Can you work these out from the model? Positions are in its coordinate system, mm. A direction names the side the tool comes from. Give positions to 0.01 mm unless a question says otherwise; leave off trailing zeros. Order: outer loops, then holes, each group sorted by start corner. A loop starts at its lowest first (then second) coordinate and runs counter-clockwise, first axis right, second up. Notation, with made-up numbers: M -16.75,-23 L 23.25,-23 A20 cw 23.25,-7 Z; hole C 28.25,-24.5 d1. An arc over 180 degrees is marked long. Use a Markdown table: item, result. Add a question column.
Autodesk Inventor part; units mm, degrees
ref_plane "YZ Plane" through (0, 0, 0) normal (1, 0, 0) x (0, 1, 0)
ref_plane "XZ Plane" through (0, 0, 0) normal (0, 1, 0) x (-1, 0, 0)
ref_plane "XY Plane" through (0, 0, 0) normal (0, 0, 1) x (1, 0, 0)
sketch "Sketch1" plane through (0, 0, 0) normal (0, 0, 1) x (1, 0, 0)
  line L0 (0, 0) -> (-184.15, 0)
  line L1 (-184.15, 0) -> (-184.15, 101.6)
  line L2 (-184.15, 101.6) -> (0, 101.6)
  line L3 (0, 101.6) -> (0, 0)
  dimension "d0" = 184.15
  dimension "d1" = 101.6
extrude "Extrusion1" add sketch "Sketch1" along normal blind 1.5875
chamfer "Chamfer1" distance 1.5875 angle 45 1 edges at (-184.15, 50.8, 0)
sketch "Sketch2" plane through (-184.15, 0, 1.5875) normal (-0.7071, 0, -0.7071) x (-0.7071, 0, 0.7071)
  line L0 (0, 101.6) -> (0, 0)
  line L1 (-2.2451, 101.6) -> (-2.2451, 0)
  line L2 (0, 101.6) -> (-2.2451, 101.6)
  line L3 (-2.2451, 0) -> (0, 0)
  point P0 (-131.3362, 0)
extrude "Extrusion2" add sketch "Sketch2" along normal blind 19.05
sketch "Sketch3" plane through (0, 0, 1.5875) normal (0, 0, 1) x (1, 0, 0)
  circle A0 centre (-19.05, 69.85) radius 2.1844
  line L0 (-184.15, 0) -> (0, 0)
  line L1 (-184.15, 101.6) -> (-184.15, 0)
  circle A1 centre (-171.45, 69.85) radius 2.1844
  point P0 (-231.8428, 57.2075)
  point P1 (-184.15, 46.6344)
  point P2 (-184.15, 42.2656)
  dimension "d9" = 4.3688
  dimension "d10" = 69.85
  dimension "d11" = 165.1
  dimension "d17" = 4.3688
  dimension "d18" = 152.4
extrude "Extrusion3" cut sketch "Sketch3" against normal blind 19.05
properties part number "frontwing"
1. On a 3-axis mill with a long thin cutter (end or side, diameter ignored), from which of +Z, -Z, +X, -X, +Y, -Y can I reach the whole of each face in a straight line? I mean faces 5 (the face through (-93, 52, 0)), 6 (the face through (-105, 0, 1)). Say none if no direction works.
2. If we section it at D-D, the plane x = -54.5: List the corners of the cut face in (y, z) for me.
3. If we section it at B-B, the plane y = 69.85: State how many separate pieces and enclosed holes the cut face has, then the cut area to 3 significant figures.
4. We'd pull the mould along Y, two halves only. Please class faces 1 (the face through (-190.79, 51.51, -5.05)), 2 (the face through (-173.632, 69.946, 0.805)), 3 (the face through (-113, 101.6, 1)), 4 (the face through (-18.042, 67.912, 0.805)): +Y half, -Y half, draft (parallel to the pull), parting line (faces both ways), or undercut.
5. I need wall thicknesses on L1, parallel to Y at x = -19.05, z = 1; L2, parallel to Z at x = -107, y = 62; L3, parallel to X at y = 46, z = -4.25. Which ranges of each line are inside material? Lowest first, please. Write a range as [from, to].
6. Will these pins go through, and if not, where does the flat tip stop? pin 1 (5 mm diameter, centred on x = -164, y = 75, fed in from -Z); pin 2 (5 mm diameter, centred on y = 20, z = -3.5, fed in from -X).
7. If we section it at A-A, the plane x = -171.45: List the corners of the cut face in (y, z) for me.
Geometry results:
| question | item | result |
|---|---|---|
| 1 | face 5 | -Z, +X, +Y, -Y |
| 1 | face 6 | +Z, -Z, +X, -X, -Y |
| 2 | outline | M 0,0 L 101.6,0 L 101.6,1.59 L 0,1.59 Z |
| 3 | separate pieces | 3 |
| 3 | enclosed holes | 0 |
| 3 | area | 320 mm^2 |
| 4 | face 1 | draft |
| 4 | face 2 | undercut |
| 4 | face 3 | +Y half |
| 4 | face 4 | undercut |
| 5 | L1 | y = [0, 67.67], [72.03, 101.6] |
| 5 | L2 | z = [0, 1.59] |
| 5 | L3 | x = [-189.99, -186.81] |
| 6 | pin 1 | stops at z = 0 |
| 6 | pin 2 | stops at x = -191.74 |
| 7 | outline | M 0,0 L 67.67,0 L 67.67,1.59 L 0,1.59 Z; M 72.03,0 L 101.6,0 L 101.6,1.59 L 72.03,1.59 Z |
